Can you work these out from the model? Positions are in its coordinate system, mm. Face numbers are marked on the shaded views. A direction names the side the tool comes from. Coordinates: 2 decimals unless noted, no trailing zeros. Loops run counter-clockwise (first coordinate to the right, second up) from the corner with the lowest first, then second, coordinate; pieces in that order, holes last.
Autodesk Inventor part; units mm, degrees
ref_plane "YZ Plane" through (0, 0, 0) normal (1, 0, 0) x (0, 1, 0)
ref_plane "XZ Plane" through (0, 0, 0) normal (0, 1, 0) x (-1, 0, 0)
ref_plane "XY Plane" through (0, 0, 0) normal (0, 0, 1) x (1, 0, 0)
sketch "스케치3" plane through (0, 0, 0) normal (0, 1, 0) x (-1, 0, 0)
  line L0 (35.7919, -14.8255) -> (14.8255, -35.7919)
  line L1 (14.8255, -35.7919) -> (-14.8255, -35.7919)
  line L2 (-14.8255, -35.7919) -> (-35.7919, -14.8255)
  line L3 (-35.7919, -14.8255) -> (-35.7919, 14.8255)
  line L4 (-35.7919, 14.8255) -> (-14.8255, 35.7919)
  line L5 (-14.8255, 35.7919) -> (14.8255, 35.7919)
  line L6 (14.8255, 35.7919) -> (35.7919, 14.8255)
  line L7 (35.7919, 14.8255) -> (35.7919, -14.8255)
  line L8 (32.5919, -13.5) -> (13.5, -32.5919)
  line L9 (13.5, -32.5919) -> (-13.5, -32.5919)
  line L10 (-13.5, -32.5919) -> (-32.5919, -13.5)
  line L11 (-32.5919, -13.5) -> (-32.5919, 13.5)
  line L12 (-32.5919, 13.5) -> (-13.5, 32.5919)
  line L13 (-13.5, 32.5919) -> (13.5, 32.5919)
  line L14 (13.5, 32.5919) -> (32.5919, 13.5)
  line L15 (32.5919, 13.5) -> (32.5919, -13.5)
  point P0 (0, 0)
  point P1 (0, 0)
  point P2 (0, 0)
  point P3 (0, 0)
  dimension "d43" = 27
  dimension "d44" = 3.2
extrude "돌출2" add sketch "스케치3" along normal blind 4.4 contours L0 L1 L2 L3 L4 L5 L6 L7 | L8 L9 L10 L11 L12 L13 L14 L15
sketch "스케치4" plane through (0, 4.4, 0) normal (0, 1, 0) x (1, 0, 0)
  line L0 (13.5, -32.5919) -> (-13.5, -32.5919)
  line L1 (-13.5, -32.5919) -> (-32.5919, -13.5)
  line L2 (-32.5919, -13.5) -> (-32.5919, 13.5)
  line L3 (-32.5919, 13.5) -> (-13.5, 32.5919)
  line L4 (-13.5, 32.5919) -> (13.5, 32.5919)
  line L5 (13.5, 32.5919) -> (32.5919, 13.5)
  line L6 (32.5919, 13.5) -> (32.5919, -13.5)
  line L7 (32.5919, -13.5) -> (13.5, -32.5919)
  line L8 (-14.1627, 34.1919) -> (14.1627, 34.1919)
  line L9 (14.1627, 34.1919) -> (34.1919, 14.1627)
  line L10 (34.1919, 14.1627) -> (34.1919, -14.1627)
  line L11 (34.1919, -14.1627) -> (14.1627, -34.1919)
  line L12 (14.1627, -34.1919) -> (-14.1627, -34.1919)
  line L13 (-14.1627, -34.1919) -> (-34.1919, -14.1627)
  line L14 (-34.1919, -14.1627) -> (-34.1919, 14.1627)
  line L15 (-34.1919, 14.1627) -> (-14.1627, 34.1919)
  line L16 (-13.3343, 32.1919) -> (13.3343, 32.1919)
  line L17 (13.3343, 32.1919) -> (32.1919, 13.3343)
  line L18 (32.1919, 13.3343) -> (32.1919, -13.3343)
  line L19 (32.1919, -13.3343) -> (13.3343, -32.1919)
  line L20 (13.3343, -32.1919) -> (-13.3343, -32.1919)
  line L21 (-13.3343, -32.1919) -> (-32.1919, -13.3343)
  line L22 (-32.1919, -13.3343) -> (-32.1919, 13.3343)
  line L23 (-32.1919, 13.3343) -> (-13.3343, 32.1919)
  line L24 (-35.7919, 14.8255) -> (-35.7919, -14.8255)
  point P0 (0, 0)
  point P1 (0, 0)
  point P2 (0, 0)
  point P3 (0, 0)
  dimension "d7" = 27
  dimension "d60" = 1.6
  dimension "d61" = 2
extrude "돌출3" cut sketch "스케치4" against normal blind 1.2 contours L0 L1 L2 L3 L4 L5 L6 L7 | L8 L9 L10 L11 L12 L13 L14 L15 | L16 L17 L18 L19 L20 L21 L22 L23
sketch "스케치5" plane through (0, 0, 0) normal (0, -1, 0) x (1, 0, 0)
  line L0 (10, 2.5) -> (20, 2.5)
  line L1 (20, 2.5) -> (20, -2.5)
  line L2 (20, -2.5) -> (10, -2.5)
  line L3 (10, -2.5) -> (10, 2.5)
  line L4 (10, 2.5) -> (20, -2.5) construction
  line L5 (20, 2.5) -> (10, -2.5) construction
  line L6 (-20, 2.5) -> (-10, 2.5)
  line L7 (-10, 2.5) -> (-10, -2.5)
  line L8 (-10, -2.5) -> (-20, -2.5)
  line L9 (-20, -2.5) -> (-20, 2.5)
  line L10 (-20, 2.5) -> (-10, -2.5) construction
  line L11 (-10, 2.5) -> (-20, -2.5) construction
  point P0 (0, 0)
  point P1 (15, 0)
  point P2 (-15, 0)
  dimension "d11" = 10
  dimension "d12" = 5
  dimension "d13" = 10
  dimension "d16" = 30
extrude "돌출4" add sketch "스케치5" along normal blind 10
sketch "스케치6" plane through (-10, 0, -2.5) normal (0, 0, -1) x (-1, 0, 0)
  circle A0 centre (5, -10) radius 5
  circle A1 centre (-25, -10) radius 5
  line L0 (-20, -10) -> (-30, -10)
  line L1 (10, -10) -> (0, -10)
  point P0 (-10, 0)
  dimension "d23" = 10
  dimension "d24" = 10
extrude "돌출5" add sketch "스케치6" against normal blind 5
sketch "스케치7" plane through (-10, 0, -2.5) normal (0, 0, -1) x (-1, 0, 0)
  circle A0 centre (5, -10) radius 1.25
  line L0 (10, 0) -> (10, -10)
  line L1 (0, 0) -> (10, 0)
  line L2 (4.7788, 0) -> (0, 0)
  circle A1 centre (-25, -10) radius 1.25
  point P0 (-10, 0)
  dimension "d27" = 2.5
  dimension "d28" = 5
  dimension "d31" = 30
extrude "돌출6" cut sketch "스케치7" against normal blind 5
sketch "스케치8" plane through (0, 0, 0) normal (0, -1, 0) x (1, 0, 0)
  circle A0 centre (0, -17.3205) radius 1.25
  line L0 (-10, 2.5) -> (-10, -2.5)
  point P0 (0, 0)
  point P1 (-10, 0)
  dimension "d38" = 2.5
  dimension "d39" = 17.3205
sketch "스케치9" plane through (0, 3.2, 0) normal (0, 1, 0) x (1, 0, 0)
  line L0 (-13.3343, 32.1919) -> (13.3343, 32.1919)
  line L1 (13.3343, 32.1919) -> (32.1919, 13.3343)
  line L2 (32.1919, 13.3343) -> (32.1919, -13.3343)
  line L3 (32.1919, -13.3343) -> (13.3343, -32.1919)
  line L4 (13.3343, -32.1919) -> (-13.3343, -32.1919)
  line L5 (-13.3343, -32.1919) -> (-32.1919, -13.3343)
  line L6 (-32.1919, -13.3343) -> (-32.1919, 13.3343)
  line L7 (-32.1919, 13.3343) -> (-13.3343, 32.1919)
  line L8 (-14.1627, 34.1919) -> (14.1627, 34.1919)
  line L9 (-12.0917, 29.1919) -> (12.0917, 29.1919)
  line L10 (12.0917, 29.1919) -> (29.1919, 12.0917)
  line L11 (29.1919, 12.0917) -> (29.1919, -12.0917)
  line L12 (29.1919, -12.0917) -> (12.0917, -29.1919)
  line L13 (12.0917, -29.1919) -> (-12.0917, -29.1919)
  line L14 (-12.0917, -29.1919) -> (-29.1919, -12.0917)
  line L15 (-29.1919, -12.0917) -> (-29.1919, 12.0917)
  line L16 (-29.1919, 12.0917) -> (-12.0917, 29.1919)
  point P0 (0, 0)
  point P1 (0, 0)
  point P2 (0, 0)
  dimension "d46" = 2
  dimension "d47" = 3
extrude "돌출8" add sketch "스케치9" along normal blind 0.6 contours L0 L1 L2 L3 L4 L5 L6 L7 | L9 L10 L11 L12 L13 L14 L15 L16
fillet "모깎기1" radius 1.2 16 edges at (-35.7919, 4.4, 0) (-25.3087, 4.4, 25.3087) (0, 4.4, 35.7919) (25.3087, 4.4, 25.3087) (35.7919, 4.4, 0) (25.3087, 4.4, -25.3087) (0, 4.4, -35.7919) (-25.3087, 4.4, -25.3087) (25.3087, 0, 25.3087) (0, 0, 35.7919) (-25.3087, 0, 25.3087) (-35.7919, 0, 0) (-25.3087, 0, -25.3087) (0, 0, -35.7919) (25.3087, 0, -25.3087) (35.7919, 0, 0)
sketch "스케치10" plane through (0, 0, 0) normal (0, -1, 0) x (1, 0, 0)
  line L0 (-20, 2.5) -> (-10, 2.5)
  line L1 (-10, -2.5) -> (-20, -2.5)
  line L2 (-20, 2.5) -> (-19, 2.5)
  line L3 (-19, 2.5) -> (-19, -2.5)
  line L4 (-19, -2.5) -> (-20, -2.5)
  line L5 (-20, -2.5) -> (-20, 2.5)
  line L6 (20, -2.5) -> (10, -2.5)
  line L7 (10, 2.5) -> (20, 2.5)
  line L8 (20, -2.5) -> (19, -2.5)
  line L9 (19, -2.5) -> (19, 2.5)
  line L10 (19, 2.5) -> (20, 2.5)
  line L11 (20, 2.5) -> (20, -2.5)
  point P0 (0, 0)
  dimension "d54" = 1
  dimension "d55" = 1
extrude "돌출9" cut sketch "스케치10" along normal blind 15
extrude "돌출10" cut sketch "스케치8" against normal blind 5
equation "\"d55\" = d54"
properties part number "OV-PAM_top_2"
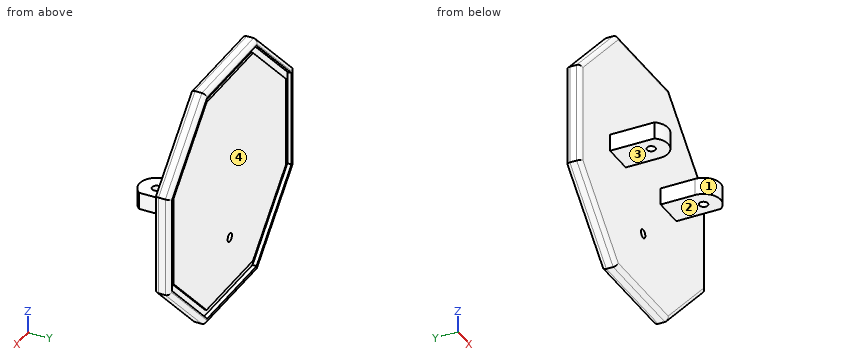
(1) If I drill on probe 1 along X at (y, z) = (-6.75, 0.5); probe 2 along Z at (x, y) = (0, 1.5); probe 3 along Y at (x, z) = (14, 6), over which ranges is the centre line in solid material (lowest first)?
Check values:
probe 1: x = -19 to -10, 10 to 19
probe 2: z = -35.79 to -18.57, -16.07 to 35.79
probe 3: y = 0 to 3.8
(2) Which directions (+Z, -Z, +X, -X, +Y, -Y) give clear straight access to the entire face, cutting with the end or side of a thin tool? Please do the marked faces 3 and 4.
Check values:
face 3: -Z, +X, -X, -Y
face 4: +Y
(3) I want a section at C-C on z = -4. Write out the boundary of the cut face in (x, y), then the cut area to 3 significant figures.
Check values:
outline: (-35.79, 1.2) arc R1.2 ccw to (-34.59, 0) - (34.59, 0) arc R1.2 ccw to (35.79, 1.2) - (35.79, 3.2) arc R1.2 ccw to (34.59, 4.4) - (34.19, 4.4) - (34.19, 3.2) - (32.19, 3.2) - (32.19, 3.8) - (-32.19, 3.8) - (-32.19, 3.2) - (-34.19, 3.2) - (-34.19, 4.4) - (-34.59, 4.4) arc R1.2 ccw to (-35.79, 3.2) - close
area: 270 mm2
(4) I want a section at B-B on x = 0. Write out the boundary of the cut face in (y, z), then the cut area to 3 significant figures.
Check values:
outline: (0, -34.59) arc R1.2 ccw to (1.2, -35.79) - (3.2, -35.79) arc R1.2 ccw to (4.4, -34.59) - (4.4, -34.19) - (3.2, -34.19) - (3.2, -32.19) - (3.8, -32.19) - (3.8, -18.57) - (0, -18.57) - close; (0, -16.07) - (3.8, -16.07) - (3.8, 32.19) - (3.2, 32.19) - (3.2, 34.19) - (4.4, 34.19) - (4.4, 34.59) arc R1.2 ccw to (3.2, 35.79) - (1.2, 35.79) arc R1.2 ccw to (0, 34.59) - close
area: 261 mm2
(5) If we mould it in two halves opening along X, with no side actions, what happens to the marked faces 1 and 2? For each: released by +X, released by -X, zero draft, split by the parting line, or undercut.
Check values:
face 1: undercut
face 2: zero draft
(6) I want a section at A-A on y = -7.5. Write out the boundary of the cut face in (x, z), then the cut area to 3 significant figures.
Check values:
outline: (-19, -2.5) - (-10, -2.5) - (-10, 2.5) - (-19, 2.5) - close; (10, -2.5) - (19, -2.5) - (19, 2.5) - (10, 2.5) - close
area: 90.0 mm2
(7) I'm going to push flat-ended pins straight in: pin 1 (6 mm diameter, centred on y = -8, z = -3.5, fed in from +X); pin 2 (4.5 mm diameter, centred on x = 15, y = -5, fed in from +Z); pin 3 (0.6 mm diameter, centred on y = 3.5, z = -1.5, fed in from -X); pin 4 (6 mm diameter, centred on x = 17.5, z = -18.5, fed in from -Y). Where does each tip first touch, or does it pass through?
Check values:
pin 1: stops at x = 19
pin 2: stops at z = 2.5
pin 3: stops at x = -35.79
pin 4: stops at y = 0
